For this review, take the finished solid that the model builds, in its own axes (mm). A direction names the side the tool comes from. Give positions to 0.01 mm unless a question says otherwise; leave off trailing zeros. Loops run counter-clockwise (first coordinate to the right, second up) from the corner with the lowest first, then second, coordinate; pieces in that order, holes last.
```python
from build123d import *

# Parameters (mm, degrees)
F0_R      = 1.75
F1_DEPTH  = 5
F2_R      = 1.75
F2_R_2    = 11.75
F3_DEPTH  = 6
F5_DEPTH  = 4
F7_DEPTH  = 4
F8_R      = 5.5
F8_R_2    = 3
F9_DEPTH  = 1.5
F10_DEPTH = 1


with BuildPart() as f1:
    # F0 (on Front) → F1 (new body)
    with BuildSketch(Plane.XZ):
        Polygon((15, 25), (-10, 25), (-10, 0), (-10, -25), (15, -25), align=None)
        with Locations((0, -15)):
            Circle(F0_R, mode=Mode.SUBTRACT)
        with Locations((0, 15)):
            Circle(F0_R, mode=Mode.SUBTRACT)
    extrude(amount=F1_DEPTH)

    # F2 (on face) → F3 (join)
    with BuildSketch(Plane.YZ.offset(15)):
        Polygon((-5, 25), (-47.3, 25), (-47.3, -25), (-5, -25), (-5, 0), align=None)
        with Locations((-41.65, -15.5)):
            Circle(F2_R, mode=Mode.SUBTRACT)
        with Locations((-10.65, -15.5)):
            Circle(F2_R, mode=Mode.SUBTRACT)
        with Locations((-41.65, 15.5)):
            Circle(F2_R, mode=Mode.SUBTRACT)
        with Locations((-26.15, 0)):
            Circle(F2_R_2, mode=Mode.SUBTRACT)
        with Locations((-10.65, 15.5)):
            Circle(F2_R, mode=Mode.SUBTRACT)
    extrude(amount=-F3_DEPTH)

    # F4 (on face) → F5 (join)
    with BuildSketch(Plane(origin=(0, 0, -25), x_dir=(1, 0, 0), z_dir=(0, 0, -1))):
        Polygon((9, 47.3), (-10, 5), (9, 5), align=None)
    extrude(amount=-F5_DEPTH)

    # F6 (on face) → F7 (join)
    with BuildSketch(Plane.XY.offset(25)):
        Polygon((-10, -5), (9, -47.3), (9, -5), align=None)
    extrude(amount=-F7_DEPTH)

    # F8 (on face) → F9 (join)
    with BuildSketch(Plane.XZ.offset(5)):
        with Locations((0, 15)):
            Circle(F8_R)
        with Locations((0, 15)):
            Circle(F8_R_2, mode=Mode.SUBTRACT)
        with Locations((0, -15)):
            Circle(F8_R)
        with Locations((0, -15)):
            Circle(F8_R_2, mode=Mode.SUBTRACT)
    extrude(amount=F9_DEPTH)

    # F10 (cut): faces of the model
    f10_faces = [f1.faces().sort_by_distance(p)[0] for p in [
        (-2.9151471863, -5, 15),
        (-2.9151471863, -5, -15),
    ]]
    extrude(f10_faces, amount=-F10_DEPTH, mode=Mode.SUBTRACT)


solid = f1.part
```
Item 1: Take a section at C-C on x = 4.5. Give the boundary of the cut face in (y, z), and give its area (3 significant figures).
Answer:
outline: (-37.28, -25) - (0, -25) - (0, 25) - (-37.28, 25) - (-37.28, 21) - (-5, 21) - (-5, 18.16) - (-6.5, 18.16) - (-6.5, 11.84) - (-5, 11.84) - (-5, -11.84) - (-6.5, -11.84) - (-6.5, -18.16) - (-5, -18.16) - (-5, -21) - (-37.28, -21) - close
area: 527 mm2
Item 2: The part is to be moulded in two halves that separate along Z. For faces 4 (the flat face through (5, -19, -25)), 5 (the cylindrical face through (12.042, -9.709, 16.976)), 6 (the flat face through (12, -47.3, 0)), say which applies: released by +Z, released by -Z, zero draft, split by the parting line, or undercut.
Answer:
face 4: released by -Z
face 5: undercut
face 6: zero draft
Item 3: For L1, parallel to Z at x = 12.85, y = -10.65; L2, parallel to Z at x = 0, y = -4.4; L3, parallel to Z at x = 0, y = -5.65, list the stretches that pass through material, from the lowest coordinate up.
Answer:
L1: z = -25 to -17.25, -13.75 to 13.75, 17.25 to 25
L2: z = -25 to -18, -12 to 12, 18 to 25
L3: z = -25 to -21, -20.5 to -18, -12 to -9.5, 9.5 to 12, 18 to 20.5, 21 to 25
Item 4: Take a section at B-B on y = -10.65. Give the boundary of the cut face in (x, z).
Answer:
outline: (-7.46, -25) - (15, -25) - (15, -17.25) - (9, -17.25) - (9, -21) - (-7.46, -21) - close; (-7.46, 21) - (9, 21) - (9, 17.25) - (15, 17.25) - (15, 25) - (-7.46, 25) - close; (9, -13.75) - (15, -13.75) - (15, 13.75) - (9, 13.75) - close
Item 5: Clearance check with flat-ended pins moving along their axes: pin 1 Ø3.5 at (x, z) = (-1, -13) entering from -Y; pin 2 Ø2 at (y, z) = (-10.65, 15.5) entering from +X; pin 3 Ø3.5 at (x, z) = (-0.5, 16) entering from -Y. State where each tip first meets the part, or that it passes through.
Answer:
pin 1: stops at y = -6.5
pin 2: passes through
pin 3: stops at y = -4
Item 6: Tool access review of faces 1 (the cylindrical face through (12.042, -9.709, -14.024)), 2 (the flat face through (4, -17, -21)), 3 (the flat face through (0, -4, -17)): name each direction out of +Z, -Z, +X, -X, +Y, -Y from which nothing blocks a thin tool from reaching the whole face with its end or side.
Answer:
face 1: +X, -X
face 2: -X, -Y
face 3: -Y
Item 7: Take a section at A-A on z = 0. Give the boundary of the cut face in (x, y).
Answer:
outline: (-10, -5) - (9, -5) - (9, -14.4) - (15, -14.4) - (15, 0) - (-10, 0) - close; (9, -47.3) - (15, -47.3) - (15, -37.9) - (9, -37.9) - close
Item 8: Take a section at D-D on y = -21. Give the boundary of the cut face in (x, z), and give its area (3 significant figures).
Answer:
outline: (-2.81, -25) - (15, -25) - (15, -10.56) - (9, -10.56) - (9, -21) - (-2.81, -21) - close; (-2.81, 21) - (9, 21) - (9, 10.56) - (15, 10.56) - (15, 25) - (-2.81, 25) - close
area: 268 mm2
